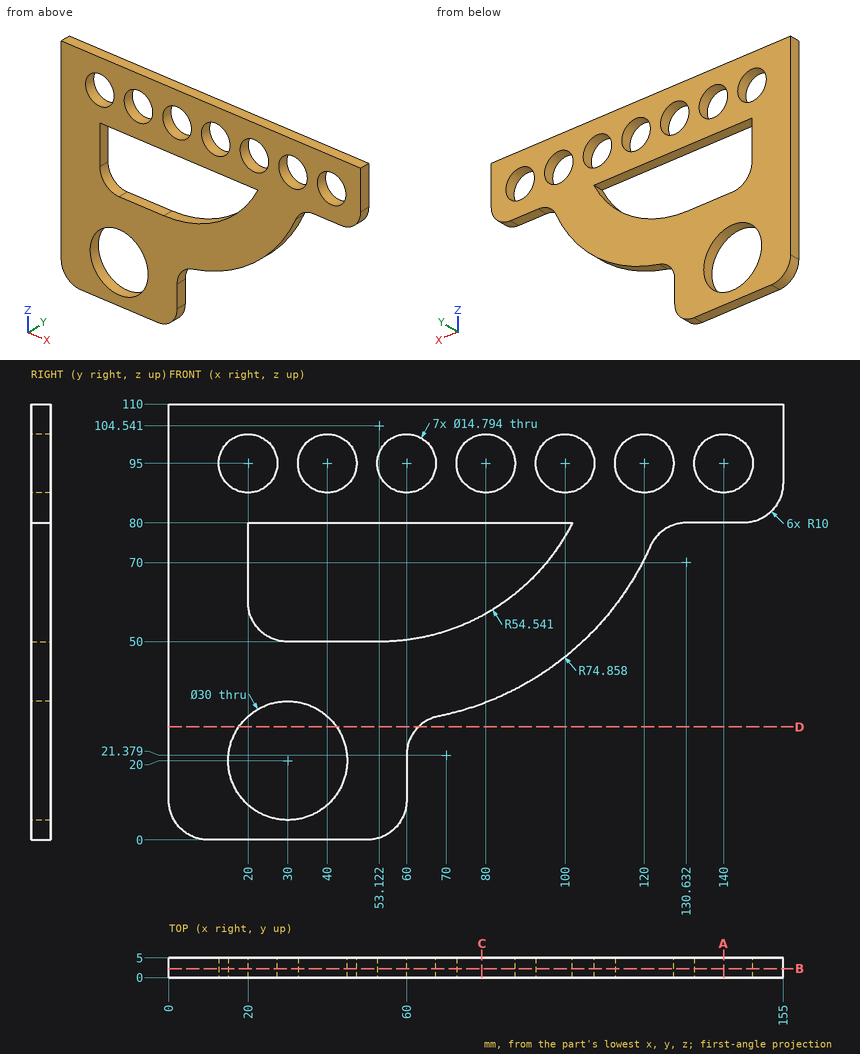
Design review of the part shown in the three views and the two pictorial views. Dimensions are in mm from the part's minimum x, y and z. Give positions to 0.01 mm unless a question says otherwise; leave off trailing zeros. Write each loop counter-clockwise with the first axis right and the second up, starting at its lowest first coordinate (ties: lowest second). Pieces come first, ordered by that corner, then holes. Notation, with made-up numbers: (2.5, 52.5) - (28.5, 52.5) arc R19 cw to (28.5, 75.5) - close; hole circle Ø11 at (-19, 59.25). An arc over 180 degrees is marked (long way). Return JSON: item names as keys, results as strings. Group by question number.
(1) To check wall thickness, follow probe 1 along Z at (x, y) = (48, 1.75); probe 2 along Z at (x, y) = (84, 2.4); probe 3 along Z at (x, y) = (30, 2.1). State the ranges of each line that lie inside material, in increasing order.
(2) We need section B-B, the plane y = 2.3. Give the number of separate pieces and of enclosed holes in the cut face, then the cut area to 3 significant figures.
(3) Insertion check: pin 1 (13.5 mm diameter, centred on x = 40, z = 95, fed in from -Y); pin 2 (1.5 mm diameter, centred on x = 95.5, y = 3, fed in from -Z) (1 decimal); pin 3 (3 mm diameter, centred on y = 2.5, z = 53, fed in from +X) (1 decimal); pin 4 (1.5 mm diameter, centred on y = 1.5, z = 72, fed in from +X). Each pin has a flat end and moves straight along its axis. Give the tip position at first contact, or say it passes through.
(4) We need section A-A, the plane x = 140. Give the boundary of the cut face in (y, z).
(5) We need section D-D, the plane z = 28.5. Give the boundary of the cut face in (x, y).
(6) We need section C-C, the plane x = 79. Give the boundary of the cut face in (y, z), then the cut area to 3 significant figures.
Reported:
{
 "1": {"probe 1": "z = 0 to 50, 80 to 110", "probe 2": "z = 36.35 to 59.58, 80 to 88.78, 101.22 to 110", "probe 3": "z = 0 to 5, 35 to 50, 80 to 110"},
 "2": {"separate pieces": "1", "enclosed holes": "9", "area": "7,730 mm2"},
 "3": {"pin 1": "passes through", "pin 2": "stops at z = 42.3", "pin 3": "stops at x = 108.8", "pin 4": "stops at x = 120.89"},
 "4": {"outline": "(0, 80) - (5, 80) - (5, 87.6) - (0, 87.6) - close; (0, 102.4) - (5, 102.4) - (5, 110) - (0, 110) - close"},
 "5": {"outline": "(0, 0) - (17.64, 0) - (17.64, 5) - (0, 5) - close; (42.36, 0) - (62.98, 0) - (62.98, 5) - (42.36, 5) - close"},
 "6": {"outline": "(0, 34.3) - (5, 34.3) - (5, 56.53) - (0, 56.53) - close; (0, 80) - (5, 80) - (5, 87.67) - (0, 87.67) - close; (0, 102.33) - (5, 102.33) - (5, 110) - (0, 110) - close", "area": "188 mm2"}
}
